Source: CAD feature listing. Evaluate the final solid. Frame: model axes, mm. Round coordinates to 2 decimals unless told otherwise and drop trailing zeros. Write each loop counter-clockwise with the first axis right and the second up, starting at its lowest first coordinate (ties: lowest second). Pieces come first, ordered by that corner, then holes. Notation, with made-up numbers: (12.5, -16) -> (42.5, -16) arc R20 ccw to (42.5, -6) -> close; hole circle Ø3 at (45.5, -7.5). An arc over 180 degrees is marked (long way). Put each result on its own line as item: value.
Autodesk Inventor part; units mm, degrees
ref_plane "YZ Plane" through (0, 0, 0) normal (1, 0, 0) x (0, 1, 0)
ref_plane "XZ Plane" through (0, 0, 0) normal (0, 1, 0) x (-1, 0, 0)
ref_plane "XY Plane" through (0, 0, 0) normal (0, 0, 1) x (1, 0, 0)
sketch "スケッチ2" plane through (0, 0, 0) normal (1, 0, 0) x (0, 1, 0)
  line L0 (-30, 10) -> (30, 10)
  line L1 (30, 10) -> (30, -10)
  line L2 (30, -10) -> (-30, -10)
  line L3 (-30, -10) -> (-30, 10)
  line L4 (-30, 10) -> (30, -10) construction
  line L5 (30, 10) -> (-30, -10) construction
  point P0 (0, 0)
  dimension "d4" = 60
  dimension "d5" = 20
extrude "押し出し2" add sketch "スケッチ2" along normal blind 10
chamfer "面取り1" distance 5 angle 45 4 edges at (10, 0, -10) (10, 30, 0) (10, 0, 10) (10, -30, 0)
properties part number "Print_Parts_U" material "PC/ABS プラスチック"
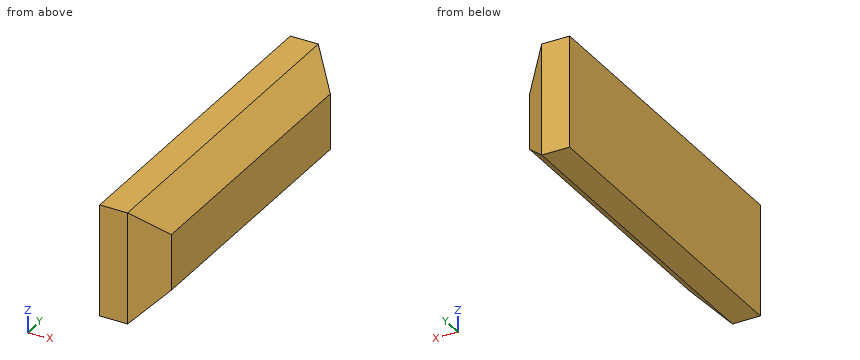
Q1. Cut plane A-A on z = -7.25. Output: boundary loops of the cut face in (x, y).
Ans:
outline: (0, -30) -> (5, -30) -> (7.75, -27.25) -> (7.75, 27.25) -> (5, 30) -> (0, 30) -> close
Q2. Pin query (flat end, axial travel): pin 1 (5 mm diameter, centred on x = 8.5, z = -5, fed in from +Y); pin 2 (5 mm diameter, centred on x = 9, y = 7, fed in from -Z). Return the tip coordinate at first contact, or that it passes through.
Ans:
pin 1: stops at y = 29
pin 2: stops at z = -8.5
Q3. Cut plane C-C on x = 7.25. Output: boundary loops of the cut face in (y, z).
Ans:
outline: (-27.75, -7.75) -> (27.75, -7.75) -> (27.75, 7.75) -> (-27.75, 7.75) -> close
Q4. Material intervals for line 1 (Y direction, x = 8.25, z = 5); line 2 (Z direction, x = 8, y = 23.5); line 3 (Y direction, x = 6.75, z = -6.5), sorted ascending. Write a range as [from, to].
Ans:
line 1: y = [-26.75, 26.75]
line 2: z = [-7, 7]
line 3: y = [-28.25, 28.25]
Q5. Cut plane B-B on y = -1.5. Output: boundary loops of the cut face in (x, z), and give its area (3 significant figures).
Ans:
outline: (0, -10) -> (5, -10) -> (10, -5) -> (10, 5) -> (5, 10) -> (0, 10) -> close
area: 175 mm^2
